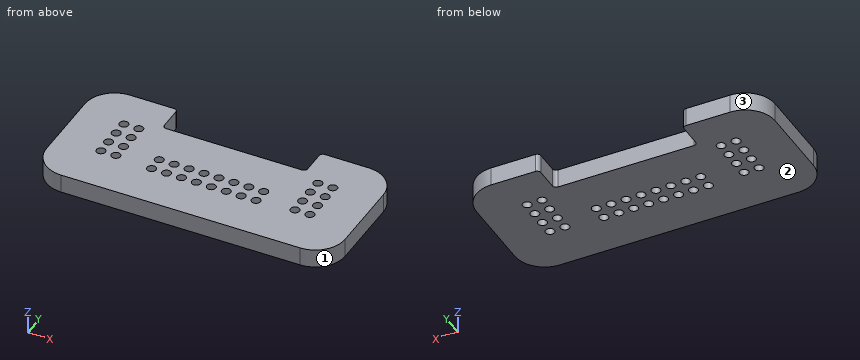
```python
from build123d import *

# Parameters (mm, degrees)
BOSS_EXTRUDE1_DEPTH = 1.6
CUT_EXTRUDE1_DEPTH  = 15.150655683
SKETCH3_R           = 0.381
CUT_EXTRUDE2_DEPTH  = 15.150655683


with BuildPart() as part:
    # Sketch1 → Boss-Extrude1 (new body)
    with BuildSketch(Plane(origin=(0, 0, -31.8411), x_dir=(-1, 0, 0), z_dir=(0, 0, -1))):
        with BuildLine():
            Line((10.16, 5.3975), (-10.16, 5.3975))
            ThreePointArc((-10.16, 5.3975), (-11.956051224, 4.653551224), (-12.7, 2.8575))
            Line((-12.7, 2.8575), (-12.7, -3.4925))
            ThreePointArc((-12.7, -3.4925), (-11.956051224, -5.288551224), (-10.16, -6.0325))
            Line((-10.16, -6.0325), (10.16, -6.0325))
            ThreePointArc((10.16, -6.0325), (11.956051224, -5.288551224), (12.7, -3.4925))
            Line((12.7, -3.4925), (12.7, 2.8575))
            ThreePointArc((12.7, 2.8575), (11.956051224, 4.653551224), (10.16, 5.3975))
        make_face()
    extrude(amount=BOSS_EXTRUDE1_DEPTH)

    # Sketch2 → Cut-Extrude1 (cut, through all)
    with BuildSketch(Plane.XY.offset(-31.8411)):
        with BuildLine():
            Line((-5.7785, 2.8575), (5.7785, 2.8575))
            ThreePointArc((5.7785, 2.8575), (6.003006403, 2.950493597), (6.096, 3.175))
            Line((6.096, 3.175), (6.096, 5.08))
            ThreePointArc((6.096, 5.08), (6.188993597, 5.304506403), (6.4135, 5.3975))
            Line((6.4135, 5.3975), (-6.4135, 5.3975))
            ThreePointArc((-6.4135, 5.3975), (-6.188993597, 5.304506403), (-6.096, 5.08))
            Line((-6.096, 5.08), (-6.096, 3.175))
            ThreePointArc((-6.096, 3.175), (-6.003006403, 2.950493597), (-5.7785, 2.8575))
        make_face()
    extrude(amount=-CUT_EXTRUDE1_DEPTH, mode=Mode.SUBTRACT)

    # Sketch3 → Cut-Extrude2 (cut, through all)
    with BuildSketch(Plane.XY.offset(-31.8411)):
        with Locations((-7.62, 1.905)):
            Circle(SKETCH3_R)
        with Locations((-8.89, 1.905)):
            Circle(SKETCH3_R)
        with Locations((-8.89, 0.635)):
            Circle(SKETCH3_R)
        with Locations((-8.89, -0.635)):
            Circle(SKETCH3_R)
        with Locations((-8.89, -1.905)):
            Circle(SKETCH3_R)
        with Locations((-7.62, 0.635)):
            Circle(SKETCH3_R)
        with Locations((-7.62, -0.635)):
            Circle(SKETCH3_R)
        with Locations((-7.62, -1.905)):
            Circle(SKETCH3_R)
        with Locations(Location((8.89, -0.635, 0), (0, 0, 180))):
            Circle(SKETCH3_R)
        with Locations(Location((8.89, -1.905, 0), (0, 0, 180))):
            Circle(SKETCH3_R)
        with Locations(Location((7.62, -1.905, 0), (0, 0, 180))):
            Circle(SKETCH3_R)
        with Locations(Location((7.62, -0.635, 0), (0, 0, 180))):
            Circle(SKETCH3_R)
        with Locations(Location((7.62, 1.905, 0), (0, 0, 180))):
            Circle(SKETCH3_R)
        with Locations(Location((7.62, 0.635, 0), (0, 0, 180))):
            Circle(SKETCH3_R)
        with Locations(Location((8.89, 0.635, 0), (0, 0, 180))):
            Circle(SKETCH3_R)
        with Locations(Location((8.89, 1.905, 0), (0, 0, 180))):
            Circle(SKETCH3_R)
        with Locations((4.445, -2.1717)):
            Circle(SKETCH3_R)
        with Locations((3.175, -2.1717)):
            Circle(SKETCH3_R)
        with Locations((1.905, -2.1717)):
            Circle(SKETCH3_R)
        with Locations((0.635, -2.1717)):
            Circle(SKETCH3_R)
        with Locations((-0.635, -2.1717)):
            Circle(SKETCH3_R)
        with Locations((-1.905, -2.1717)):
            Circle(SKETCH3_R)
        with Locations((-3.175, -2.1717)):
            Circle(SKETCH3_R)
        with Locations((-4.445, -2.1717)):
            Circle(SKETCH3_R)
        with Locations((3.175, -0.9017)):
            Circle(SKETCH3_R)
        with Locations((1.905, -0.9017)):
            Circle(SKETCH3_R)
        with Locations((0.635, -0.9017)):
            Circle(SKETCH3_R)
        with Locations((-0.635, -0.9017)):
            Circle(SKETCH3_R)
        with Locations((-1.905, -0.9017)):
            Circle(SKETCH3_R)
        with Locations((-3.175, -0.9017)):
            Circle(SKETCH3_R)
        with Locations((-4.445, -0.9017)):
            Circle(SKETCH3_R)
        with Locations((4.445, -0.9017)):
            Circle(SKETCH3_R)
    extrude(amount=-CUT_EXTRUDE2_DEPTH, mode=Mode.SUBTRACT)


solid = part.part
```
Input: part model. Units: mm. Frame: model coordinates. Face numbers are marked on the shaded views. Coordinates: 2 decimals unless noted, no trailing zeros. Loops run counter-clockwise (first coordinate to the right, second up) from the corner with the lowest first, then second, coordinate; pieces in that order, holes last. Notation, with made-up numbers: (-27, 21.25) - (21, 21.25) arc R23 cw to (21, 57.25) - close; hole circle Ø6 at (-36, 14). An arc over 180 degrees is marked (long way). Answer in a Markdown table with one row per item.
(1) Pin query (flat end, axial travel): P1, Ø0.5, axis at y = 4, z = -33, coming from the +X side. Return the tip coordinate at first contact, or that it passes through.
Model answer:
| item | result |
|---|---|
| P1 | stops at x = 12.54 |
(2) Cut plane B-B on y = 3.5. Output: boundary loops of the cut face in (x, z).
Model answer:
| item | result |
|---|---|
| outline | (-12.62, -33.44) - (-6.1, -33.44) - (-6.1, -31.84) - (-12.62, -31.84) - close; (6.1, -33.44) - (12.62, -33.44) - (12.62, -31.84) - (6.1, -31.84) - close |
(3) Cut plane D-D on y = -5.5. Output: boundary loops of the cut face in (x, z), plus the area to 3 significant figures.
Model answer:
| item | result |
|---|---|
| outline | (-11.72, -33.44) - (11.72, -33.44) - (11.72, -31.84) - (-11.72, -31.84) - close |
| area | 37.5 mm² |
(4) Mould query, pull axis Y, two halves, no side actions, for the marked faces 1, 2 and 3. Classes: pulls with the +Y half, pulls with the -Y half, needs draft (parallel to the pull), parting line crosses it, or undercut.
Model answer:
| item | result |
|---|---|
| face 1 | pulls with the -Y half |
| face 2 | needs draft |
| face 3 | pulls with the +Y half |
(5) Cut plane A-A on x = -7.62. Output: boundary loops of the cut face in (y, z), plus the area to 3 significant figures.
Model answer:
| item | result |
|---|---|
| outline | (-6.03, -33.44) - (-2.29, -33.44) - (-2.29, -31.84) - (-6.03, -31.84) - close; (-1.52, -33.44) - (-1.02, -33.44) - (-1.02, -31.84) - (-1.52, -31.84) - close; (-0.25, -33.44) - (0.25, -33.44) - (0.25, -31.84) - (-0.25, -31.84) - close; (1.02, -33.44) - (1.52, -33.44) - (1.52, -31.84) - (1.02, -31.84) - close; (2.29, -33.44) - (5.4, -33.44) - (5.4, -31.84) - (2.29, -31.84) - close |
| area | 13.4 mm² |
(6) Cut plane C-C on z = -32.4. Count the separate pieces of the cut face and the enclosed holes in it, plus the area to 3 significant figures.
Model answer:
| item | result |
|---|---|
| separate pieces | 1 |
| enclosed holes | 32 |
| area | 239 mm² |
(7) Material intervals for L1, parallel to Y at x = 7.62, z = -32.4; L2, parallel to Y at x = 3.5, z = -32.05; L3, parallel to X at y = 1.75, z = -32.45, sorted ascending. Write a range as from..to.
Model answer:
| item | result |
|---|---|
| L1 | y = -6.03..-2.29, -1.52..-1.02, -0.25..0.25, 1.02..1.52, 2.29..5.4 |
| L2 | y = -6.03..-2.37, -1.97..-1.1, -0.7..2.86 |
| L3 | x = -12.7..-9.24, -8.54..-7.97, -7.27..7.27, 7.97..8.54, 9.24..12.7 |
